Can you work these out from the model? Positions are in its coordinate system, mm. Face numbers are marked on the shaded views. Give positions to 0.01 mm unless a question says otherwise; leave off trailing zeros. Order: outer loops, then holes, each group sorted by start corner. A loop starts at its lowest first (then second) coordinate and runs counter-clockwise, first axis right, second up.
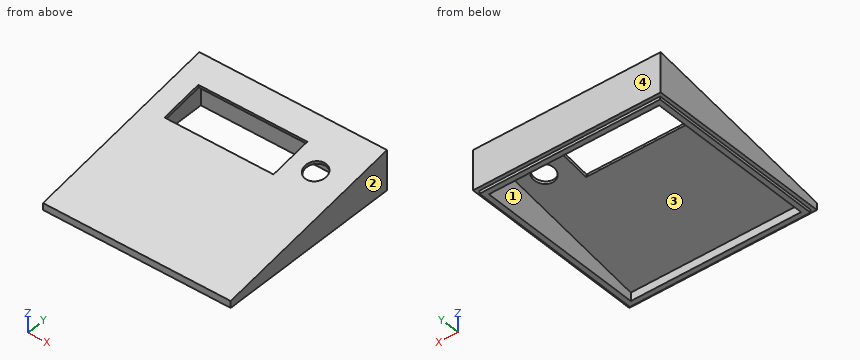
```python
from build123d import *

# Parameters (mm, degrees)
SKETCH1_W           = 87.8
SKETCH1_H           = 87.8
BOSS_EXTRUDE1_DEPTH = 20
SKETCH2_W           = 87.8
SKETCH2_H           = 87.8
SKETCH2_W_2         = 84.5
SKETCH2_H_2         = 84.5
CUT_EXTRUDE1_DEPTH  = 1.4
CUT_EXTRUDE2_DEPTH  = 126.768358501
CUT_EXTRUDE3_REACH  = 127.768
SKETCH4_W           = 79.7
SKETCH4_H           = 79.7
SKETCH5_R           = 5
SKETCH5_W           = 51
SKETCH5_H           = 19.304
CUT_EXTRUDE4_DEPTH  = 126.686719868


with BuildPart() as part:
    # Sketch1 → Boss-Extrude1 (new body)
    with BuildSketch(Plane.XY):
        with Locations((43.9, 43.9)):
            Rectangle(SKETCH1_W, SKETCH1_H)
    extrude(amount=BOSS_EXTRUDE1_DEPTH)

    # Sketch2 → Cut-Extrude1 (cut)
    with BuildSketch(Plane(origin=(0, 0, 0), x_dir=(-1, 0, 0), z_dir=(0, 0, -1))):
        with Locations((-43.9, 43.9)):
            Rectangle(SKETCH2_W, SKETCH2_H)
        with Locations((-43.9, 43.9)):
            Rectangle(SKETCH2_W_2, SKETCH2_H_2, mode=Mode.SUBTRACT)
    extrude(amount=-CUT_EXTRUDE1_DEPTH, mode=Mode.SUBTRACT)

    # Sketch3 → Cut-Extrude2 (cut, through all)
    with BuildSketch(Plane(origin=(87.8, 0, 0), x_dir=(0, 0, -1), z_dir=(1, 0, 0))):
        Polygon((-20, 87.8), (-4.6, 0), (-20, 0), align=None)
    extrude(amount=-CUT_EXTRUDE2_DEPTH, mode=Mode.SUBTRACT)

    # Cut-Extrude3: up to this plane
    cut_extrude3_end = Plane(origin=(0, 88.041865807, 18.621050787), z_dir=(0, 0.17276129088861056, -0.9849637233779227))
    # Sketch4 → Cut-Extrude3 (cut, up to the surface)
    with BuildSketch(Plane(origin=(0, 0, 0), x_dir=(-1, 0, 0), z_dir=(0, 0, -1)), mode=Mode.PRIVATE) as cut_extrude3_sk1:
        with Locations((-43.9, 43.9)):
            Rectangle(SKETCH4_W, SKETCH4_H)
    cut_extrude3_tool1 = split(extrude(cut_extrude3_sk1.sketch, amount=-CUT_EXTRUDE3_REACH, mode=Mode.PRIVATE), bisect_by=cut_extrude3_end, keep=Keep.BOTH, mode=Mode.PRIVATE)
    add(cut_extrude3_tool1.solids().sort_by_distance((43.9, 43.9, 0))[0], mode=Mode.SUBTRACT)

    # Sketch5 → Cut-Extrude4 (cut, through all)
    with BuildSketch(Plane(origin=(0, -0.78275258, 4.462706267), x_dir=(1, 0, 0), z_dir=(0, -0.1727612908886106, 0.9849637233779227))):
        with Locations(Location((72.8, 67.524905437, 0), (0, 0, 270))):
            Circle(SKETCH5_R)
        with Locations((35.5, 67.524905437)):
            Rectangle(SKETCH5_W, SKETCH5_H)
    extrude(amount=-CUT_EXTRUDE4_DEPTH, mode=Mode.SUBTRACT)


solid = part.part
```
1) I'm going to push flat-ended pins straight in: pin 1 Ø1.5 at (x, y) = (19.5, 34.5) entering from -Z; pin 2 Ø0.7 at (x, z) = (56.5, 0.5) entering from -Y; pin 3 Ø0.7 at (x, z) = (48, 0.5) entering from +Y. Where does each tip first touch, or does it pass through?
2) Suppose I cut it at D-D (y = 66). Give the number of separate pieces and of enclosed holes in the cut face, and give its area (3 significant figures).
3) Suppose I cut it at B-B (z = 6). Please give me the cut outline in (x, y), and give its area (3 significant figures).
4) Suppose I cut it at C-C (y = 21.5). Please give me the cut outline in (x, z), and give its area (3 significant figures).
5) Suppose I cut it at A-A (x = 17). Please give me the cut outline in (y, z), and give its area (3 significant figures).
6) If I drill on line 1 (Y direction, x = 23.5, z = 1); line 2 (X direction, y = 50.5, z = 11), over which ranges is the centre line in solid material (lowest first)?
7) We'd pull the mould along Y, two halves only. Please class the marked faces 1, 2, 3 and 4: +Y half, -Y half, draft (parallel to the pull), parting line (faces both ways), or undercut.
Results:
1. pin 1: stops at z = 9.1
1. pin 2: stops at y = 1.65
1. pin 3: stops at y = 86.15
2. separate pieces: 3
2. enclosed holes: 0
2. area: 153 mm2
3. outline: (0, 7.98) - (87.8, 7.98) - (87.8, 87.8) - (0, 87.8) - close; hole (4.05, 16.09) - (83.75, 16.09) - (83.75, 83.75) - (4.05, 83.75) - close
3. area: 1,620 mm2
4. outline: (0, 1.4) - (1.65, 1.4) - (1.65, 0) - (4.05, 0) - (4.05, 6.95) - (83.75, 6.95) - (83.75, 0) - (86.15, 0) - (86.15, 1.4) - (87.8, 1.4) - (87.8, 8.37) - (0, 8.37) - close
4. area: 176 mm2
5. outline: (0, 1.4) - (1.65, 1.4) - (1.65, 0) - (4.05, 0) - (4.05, 3.89) - (56.46, 13.08) - (56.22, 14.46) - (0, 4.6) - close; (75.23, 17.8) - (75.48, 16.42) - (83.75, 17.87) - (83.75, 0) - (86.15, 0) - (86.15, 1.4) - (87.8, 1.4) - (87.8, 20) - close
5. area: 181 mm2
6. line 1: y = 1.65 to 4.05, 83.75 to 86.15
6. line 2: x = 0 to 4.05, 83.75 to 87.8
7. face 1: undercut
7. face 2: draft
7. face 3: undercut
7. face 4: +Y half
